```python
from build123d import *

# Parameters (mm, degrees)
F0_W     = 80.75
F0_H     = 10.75
F1_DEPTH = 48
F2_W     = 75.5
F2_H     = 5.75
F3_DEPTH = 15
F4_SIZE2 = 8.798818
F4_SIZE  = 5.08


with BuildPart() as f1:
    # F0 (on Top) → F1 (new body)
    with BuildSketch(Plane.XY):
        Rectangle(F0_W, F0_H)
    extrude(amount=F1_DEPTH)

    # F2 (on face) → F3 (cut)
    with BuildSketch(Plane(origin=(0, 0, 0), x_dir=(1, 0, 0), z_dir=(0, 0, -1))):
        Rectangle(F2_W, F2_H)
    extrude(amount=-F3_DEPTH, mode=Mode.SUBTRACT)

    # F4
    f4_edges = [f1.edges().sort_by_distance(p)[0] for p in [
        (0, -5.375, 48),
    ]]
    chamfer(f4_edges, length=F4_SIZE, length2=F4_SIZE2)


solid = f1.part
```
The model under review builds one solid part; all positions refer to its coordinate system, in mm. A direction names the side the tool comes from. Coordinates: 2 decimals unless noted, no trailing zeros. Order: outer loops, then holes, each group sorted by start corner. A loop starts at its lowest first (then second) coordinate and runs counter-clockwise, first axis right, second up. Notation, with made-up numbers: (2.25, 19.5) -> (11.25, 19.5) arc R22 cw to (11.25, 47.5) -> close; hole circle Ø8 at (68, -26.5). An arc over 180 degrees is marked (long way). Answer in a Markdown table with one row per item. Add a question column.
Item 1: Mouldability with a two-part tool opening along X and no side actions: class faces 3 (the flat face through (-1, 0, 15)), 4 (the flat face through (-40.375, 0, 24)), 5 (the flat face through (-1, 4, 48)) as +X half, -X half, draft (parallel to the pull), parting line (faces both ways), or undercut.
Item 2: To check wall thickness, follow probe 1 along X at (y, z) = (0.25, 5.5) (3 decimals); probe 2 along Y at (x, z) = (-19, 14.5) (3 decimals); probe 3 along Z at (x, y) = (-27, 0.25). State the ranges of each line that lie inside material, in increasing order.
Item 3: We need section B-B on x = 18. Write out the cut boundary in (y, z) (3 decimals), plus the area to 3 significant figures.
Item 4: We need section C-C on y = 1.75. Write out the cut boundary in (x, z) (3 decimals), plus the area to 3 significant figures.
Item 5: We need section A-A on z = 8. Write out the cut boundary in (x, y) (3 decimals), plus the area to 3 significant figures.
Item 6: We need section D-D on y = -4.25. Write out the cut boundary in (x, z) (3 decimals), plus the area to 3 significant figures.
Item 7: Machinability: for faces 1 (the flat face through (-1, 2.875, 7)), 2 (the flat face through (-1, 5.375, 24)), which of the approach directions +Z, -Z, +X, -X, +Y, -Y give a long, thin tool a straight path to every point of the face, cutting with its end or side? Answer none if there is none.
Final values:
| question | item | result |
|---|---|---|
| 1 | face 3 | undercut |
| 1 | face 4 | -X half |
| 1 | face 5 | draft |
| 2 | probe 1 | x = -40.375 to -37.75, 37.75 to 40.375 |
| 2 | probe 2 | y = -5.375 to -2.875, 2.875 to 5.375 |
| 2 | probe 3 | z = 15 to 46.17 |
| 3 | outline | (-5.375, 0) -> (-2.875, 0) -> (-2.875, 15) -> (2.875, 15) -> (2.875, 0) -> (5.375, 0) -> (5.375, 48) -> (3.424, 48) -> (-5.375, 42.92) -> close |
| 3 | area | 407 mm2 |
| 4 | outline | (-40.375, 0) -> (-37.75, 0) -> (-37.75, 15) -> (37.75, 15) -> (37.75, 0) -> (40.375, 0) -> (40.375, 47.034) -> (-40.375, 47.034) -> close |
| 4 | area | 2,670 mm2 |
| 5 | outline | (-40.375, -5.375) -> (40.375, -5.375) -> (40.375, 5.375) -> (-40.375, 5.375) -> close; hole (-37.75, -2.875) -> (37.75, -2.875) -> (37.75, 2.875) -> (-37.75, 2.875) -> close |
| 5 | area | 434 mm2 |
| 6 | outline | (-40.375, 0) -> (40.375, 0) -> (40.375, 43.57) -> (-40.375, 43.57) -> close |
| 6 | area | 3,520 mm2 |
| 7 | face 1 | -Z |
| 7 | face 2 | +Z, -Z, +X, -X, +Y |
